from build123d import *

# Parameters (mm, degrees)
SKETCH_1_R             = 8
SM_BASE_FLANGE_1_DEPTH = 4


# Sheet-metal steps are written as plain solids
with BuildPart() as part:
    # Sketch 1 → Базовая кромка1 (new body)
    with BuildSketch(Plane(origin=(0, 0, 0), x_dir=(0, 0, -1), z_dir=(1, 0, 0))):
        with BuildLine():
            Line((-161.097577427, 311.348014413), (15.777028295, 170.442439889))
            ThreePointArc((15.777028295, 170.442439889), (21.027340211, 152.992649587), (6.535875187, 141.944645322))
            ThreePointArc((6.535875187, 141.944645322), (-8.680633455, 133.794281683), (-11.883786143, 116.832254223))
            Line((-11.883786143, 116.832254223), (17.41991669, 6.481832542))
            ThreePointArc((17.41991669, 6.481832542), (17.268656425, 5.060014039), (16.206724964, 4.102543887))
            Line((16.206724964, 4.102543887), (15.1830333, 3.707647452))
            ThreePointArc((15.1830333, 3.707647452), (13.65244827, 3.7453323), (12.596997586, 4.854446603))
            ThreePointArc((12.596997586, 4.854446603), (-4.858743487, 12.595340874), (-12.593682696, -4.863039806))
            ThreePointArc((-12.593682696, -4.863039806), (-12.630845419, -6.393637603), (-13.739599615, -7.449466574))
            Line((-13.739599615, -7.449466574), (-14.763291279, -7.844363009))
            ThreePointArc((-14.763291279, -7.844363009), (-16.19312815, -7.848110442), (-17.26006382, -6.896219798))
            Line((-17.26006382, -6.896219798), (-182.737745394, 313.474626916))
            ThreePointArc((-182.737745394, 313.474626916), (-171.603404739, 315.609160958), (-161.097577427, 311.348014413))
        make_face()
        with Locations((5.807559646, 157.928060366)):
            Circle(SKETCH_1_R, mode=Mode.SUBTRACT)
    extrude(amount=SM_BASE_FLANGE_1_DEPTH)


solid = part.part
Build history of the part. All positions in model axes, mm. A direction names the side the tool comes from. Give positions to 0.01 mm unless a question says otherwise; leave off trailing zeros. Loops run counter-clockwise (first coordinate to the right, second up) from the corner with the lowest first, then second, coordinate; pieces in that order, holes last. Notation, with made-up numbers: (-38, 26) - (-3, 26) arc R29 ccw to (-3, 49) - close; hole circle Ø10 at (-24.5, 60.5). An arc over 180 degrees is marked (long way). Write item = value, one per line. Start each with the question number.
1) Pull direction Y, two halves, no side cores. Call faces 1 (the cylindrical face through (1.97, 165.86, -4.77)), 2 (the cylindrical face through (1.972, 133.995, 8.532)), 3 (the flat face through (1.972, 151.047, 98.841)), 4 (the flat face through (4, 167, 65)): +Y half, -Y half, draft (parallel to the pull), parting line (faces both ways), or undercut.
2) Drop flat-ended pins along their axis: pin 1 Ø1.5 at (x, z) = (1.5, 55) entering from -Y; pin 2 Ø1.5 at (x, z) = (0.5, 25.5) entering from -Y. Give the stop position or say it passes through.
3) Band-saw the part on B-B on x = 3.2. Give the cut face in (y, z).
4) Band-saw the part on A-A on z = -2. Give the cut face in (x, y), plus the area to 3 significant figures.
5) Tool access for faces 5 (the flat face through (1.972, 241.882, 73.898)), 6 (the flat face through (1.972, 62.429, -2.563)): list every direction of +Z, -Z, +X, -X, +Y, -Y with a clear straight run to the whole face (end or side of a thin tool).
6) Band-saw the part on C-C on y = 94.5. Give the cut face in (x, z), plus the area to 3 significant figures.
7) Probe probe 1 along Z at (x, y) = (0.35, 12); probe 2 along Z at (x, y) = (0.95, 32.5); probe 3 along Y at (x, z) = (3.7, 69.5). List the from-to ranges inside material, lowest first. Write a range as from..to.
8) Band-saw the part on D-D on z = 156. Give the cut face in (x, y), plus the area to 3 significant figures.
Final values:
q1.face_1 = undercut
q1.face_2 = undercut
q1.face_3 = -Y half
q1.face_4 = draft
q2.pin_1 = 64.72
q2.pin_2 = 7.6
q3.outline = (-7.84, 14.76) - (-7.45, 13.74) arc R2 ccw to (-4.86, 12.59) arc R13.5 cw to (4.85, -12.6) arc R2 ccw to (3.71, -15.18) - (4.1, -16.21) arc R2 ccw to (6.48, -17.42) - (116.83, 11.88) arc R20 cw to (141.94, -6.54) arc R16 ccw to (170.44, -15.78) - (311.35, 161.1) arc R20 ccw to (313.47, 182.74) - (-6.9, 17.26) arc R2 ccw to start; hole circle Ø16 at (157.93, -5.81)
q4.outline = (0, 13.35) - (4, 13.35) - (4, 64.55) - (0, 64.55) - close; (0, 141.21) - (4, 141.21) - (4, 150.89) - (0, 150.89) - close; (0, 164.96) - (4, 164.96) - (4, 181.42) - (0, 181.42) - close
q4.area = 309 mm²
q5.face_5 = -Z, +X, -X, +Y
q5.face_6 = -Z, +X, -X
q6.outline = (0, 5.95) - (4, 5.95) - (4, 69.63) - (0, 69.63) - close
q6.area = 255 mm²
q7.probe_1 = -15.95..-6.18, 6.18..27.02
q7.probe_2 = -10.51..37.61
q7.probe_3 = 94.24..238.38
q8.outline = (0, 261.71) - (4, 261.71) - (4, 307.29) - (0, 307.29) - close
q8.area = 182 mm²
